Autodesk Inventor part; units mm, degrees
ref_plane "YZ Plane" through (0, 0, 0) normal (1, 0, 0) x (0, 1, 0)
ref_plane "XY Plane" through (0, 0, 0) normal (0, 0, 1) x (1, 0, 0)
sketch "Sketch1" plane through (0, 0, 0) normal (0, 0, 1) x (1, 0, 0)
  line L0 (-17.25, -31.85) -> (4.85, -31.85)
  line L1 (4.85, -31.85) -> (4.85, 0)
  arc A0 (4.85, 0) -> (0, 4.85) centre (0, 0) ccw
  line L2 (0, 4.85) -> (-12.4, 4.85)
  arc A1 (-12.4, 4.85) -> (-17.25, 0) centre (-12.4, 0) ccw
  line L3 (-17.25, 0) -> (-17.25, -31.85)
  circle A2 centre (-6.2, -6.5) radius 2.75
  circle A3 centre (-6.2, -17.15) radius 1.95
  arc A4 (1.9991, -27.9755) -> (1.0928, -27.0978) centre (2.55, -26.5) ccw
  arc A5 (1.0928, -27.0978) -> (1.9991, -27.9755) centre (-0.065, -29.2) ccw
  arc A6 (-13.4928, -27.0978) -> (-14.3991, -27.9755) centre (-14.95, -26.5) ccw
  arc A7 (-14.3991, -27.9755) -> (-13.4928, -27.0978) centre (-12.335, -29.2) ccw
  line L4 (9.85, -61.85) -> (-22.25, -61.85)
  line L5 (-22.25, -61.85) -> (-22.25, -21.85)
  line L6 (-22.25, -21.85) -> (9.85, -21.85)
  line L7 (9.85, -21.85) -> (9.85, -61.85)
  circle A8 centre (2.55, -26.5) radius 1.575
  circle A9 centre (-14.95, -26.5) radius 1.575
  point P0 (0, 0)
  point P1 (1.0928, -27.0978)
  point P2 (1.9991, -27.9755)
  point P3 (-17.25, -21.85)
  point P4 (4.85, -21.85)
  dimension "d2" = 5
  dimension "d3" = 5
  dimension "d12" = 10
  dimension "d13" = 40
extrude "Extrusion2" add sketch "Sketch1" along normal blind 5 contours L3 L6 L1 L0 | L0 L1 L6 L7 L4 L5 L3 | A5 A8 | A7 A9
sketch "Sketch2" plane through (0, 0, 0) normal (0, 0, -1) x (-1, 0, 0)
  line L0 (22.25, -21.85) -> (22.25, -61.85)
  line L1 (22.25, -61.85) -> (18.25, -61.85)
  line L2 (18.25, -61.85) -> (18.25, -21.85)
  line L3 (18.25, -21.85) -> (22.25, -21.85)
  line L4 (22.25, -21.85) -> (22.25, -61.85)
  line L5 (-9.85, -61.85) -> (-9.85, -21.85)
  line L6 (-9.85, -21.85) -> (22.25, -21.85)
  line L7 (-9.85, -61.85) -> (-5.85, -61.85)
  line L8 (-5.85, -61.85) -> (-5.85, -21.85)
  line L9 (-5.85, -21.85) -> (-9.85, -21.85)
  line L10 (-9.85, -21.85) -> (-9.85, -61.85)
  point P0 (0, 0)
  point P1 (-4.85, -21.85)
  point P2 (17.25, -21.85)
  point P3 (-9.85, -21.85)
  dimension "d8" = 4
  dimension "d9" = 4
extrude "Extrusion3" add sketch "Sketch2" along normal blind 20
sketch "Sketch3" plane through (0, 0, -20) normal (0, 0, -1) x (-1, 0, 0)
  circle A0 centre (-2.55, -26.5) radius 1.575
  circle A1 centre (14.95, -26.5) radius 1.575
  circle A2 centre (6.2, -6.5) radius 2.95
  line L0 (-43.9339, 5.041) -> (56.0661, 5.041)
  line L1 (-23.9339, -29.6) -> (-43.9339, 5.041)
  line L2 (36.0661, -29.6) -> (-23.9339, -29.6)
  line L3 (56.0661, 5.041) -> (36.0661, -29.6)
  line L4 (22.25, -61.85) -> (-9.85, -61.85)
  line L5 (-9.85, -61.85) -> (-9.85, -21.85)
  line L6 (22.25, -61.85) -> (-9.85, -61.85)
  line L7 (-9.85, -61.85) -> (-9.85, -30.6)
  line L8 (-9.85, -30.6) -> (22.25, -30.6)
  line L9 (22.25, -30.6) -> (22.25, -61.85)
  point P0 (0, 0)
  dimension "d14" = 1
extrude "Extrusion4" add sketch "Sketch3" along normal blind 5 contours L8 L9 L4 L5
sketch "Sketch4" plane through (0, 0, 5) normal (0, 0, 1) x (1, 0, 0)
  circle A0 centre (-6.2, -46.85) radius 11.05
  line L0 (-22.25, -21.85) -> (-22.25, -61.85)
  line L1 (-22.25, -61.85) -> (9.85, -61.85)
  point P0 (0, 0)
  dimension "d17" = 22.1
  dimension "d18" = 16.05
  dimension "d19" = 15
extrude "Extrusion5" cut sketch "Sketch4" against normal up to surface (5 mm away)
sketch "Sketch5" plane through (0, 0, -25) normal (0, 0, -1) x (-1, 0, 0)
  circle A0 centre (6.2, -46.85) radius 4.508
  circle A1 centre (6.2, -46.85) radius 15
  line L0 (22.25, -21.85) -> (22.25, -61.85)
  line L1 (22.25, -46.85) -> (-9.85, -46.85)
  line L2 (-9.85, -61.85) -> (-9.85, -21.85)
  line L3 (22.25, -46.85) -> (22.25, -61.85)
  line L4 (22.25, -61.85) -> (-9.85, -61.85)
  line L5 (-9.85, -46.85) -> (-9.85, -61.85)
  point P0 (0, 0)
  point P1 (6.2, -61.85)
  point P2 (21.2, -46.85)
  point P3 (-8.8, -46.85)
  dimension "d22" = 30
extrude "Extrusion6" cut sketch "Sketch5" against normal up to surface (30 mm away) contours L1 L0 L4 A1 | A1 L4 L2 L1
ref_plane "Work Plane1" through (-6.2, -61.85, -25) normal (0, 1, 0) x (-1, 0, 0)
sketch "Sketch6" plane through (-6.2, -61.85, -25) normal (0, 1, 0) x (-1, 0, 0)
  line L0 (-15, 0) -> (15, 0)
  line L1 (-15, 0) -> (-15, 30)
  line L2 (15, 30) -> (-15, 30)
  line L3 (15, 0) -> (15, 30)
  line L4 (12.05, 5) -> (-12.05, 5)
  line L5 (12.05, 25) -> (12.05, 5)
  line L6 (-12.05, 25) -> (12.05, 25)
  line L7 (-12.05, 5) -> (-12.05, 25)
  line L8 (-12.05, 25) -> (12.05, 25)
  line L9 (12.05, 25) -> (12.05, 26.5)
  line L10 (12.05, 26.5) -> (-12.05, 26.5)
  line L11 (-12.05, 26.5) -> (-12.05, 25)
  line L12 (-12.05, 5) -> (12.05, 5)
  line L13 (12.05, 5) -> (12.05, 3.5)
  line L14 (12.05, 3.5) -> (-12.05, 3.5)
  line L15 (-12.05, 3.5) -> (-12.05, 5)
  point P0 (-6.2, 25)
  dimension "d25" = 1.5
  dimension "d26" = 1.5
extrude "Extrusion7" cut sketch "Sketch6" along normal up to surface (40 mm away) contours L13 L14 L15 L4 | L6 L11 L10 L9
properties part number "arm1"
The listing builds one solid part. Answer for the finished solid, in the listing's coordinates (mm). A direction names the side the tool comes from. Give positions to 0.01 mm unless a question says otherwise; leave off trailing zeros. Write each loop counter-clockwise with the first axis right and the second up, starting at its lowest first coordinate (ties: lowest second). Pieces come first, ordered by that corner, then holes. Notation, with made-up numbers: M 40,2 L 97,2 A14 ccw 97,19 Z; hole C 81.5,52.25 d6. An arc over 180 degrees is marked long. Write each question's results on one line, items separated by ' | '.
Q1. Section C-C, the plane x = -15 is taken. Write down the section's boundary in (y, z), then the cut area to 3 significant figures.
Output values:
outline: M -59,-25 L -30.6,-25 L -30.6,-21.5 L -59,-21.5 Z; M -59,1.5 L -53.53,1.5 L -53.53,5 L -59,5 Z; M -40.17,1.5 L -28.07,1.5 L -28.07,5 L -40.17,5 Z; M -24.93,1.5 L -21.85,1.5 L -21.85,5 L -24.93,5 Z | area: 172 mm2
Q2. Section A-A, the plane z = -14.5 is taken. Write down the section's boundary in (x, y).
Output values:
outline: M -22.25,-46.85 L -21.2,-46.85 A15 ccw -18.25,-55.78 L -18.25,-21.85 L -22.25,-21.85 Z; M 5.85,-55.78 A15 ccw 8.8,-46.85 L 9.85,-46.85 L 9.85,-21.85 L 5.85,-21.85 Z
Q3. Section B-B, the plane x = -6.2 is taken. Write down the section's boundary in (y, z).
Output values:
outline: M -61.85,-25 L -30.6,-25 L -30.6,-21.5 L -61.85,-21.5 Z; M -61.85,1.5 L -57.9,1.5 L -57.9,5 L -61.85,5 Z; M -35.8,1.5 L -21.85,1.5 L -21.85,5 L -35.8,5 Z
Q4. Consider L1, parallel to X at y = -35, z = -17.75; L2, parallel to Y at x = -6.2, z = 3.5; L3, parallel to Z at x = -10, y = -32.5. Determine where each line is inside the solid, lowest interval first. Write a range as from..to.
Output values:
L1: -22.25..-18.25, 5.85..9.85 | L2: -61.85..-57.9, -35.8..-21.85 | L3: -25..-21.5, 1.5..5
Q5. Section D-D, the plane y = -46 is taken. Write down the section's boundary in (x, z).
Output values:
outline: M -22.25,-25 L 9.85,-25 L 9.85,5 L 4.82,5 L 4.82,1.5 L 5.85,1.5 L 5.85,-21.5 L -18.25,-21.5 L -18.25,1.5 L -17.22,1.5 L -17.22,5 L -22.25,5 Z
Q6. For a pull along Y with two mould halves and no side action, classify faces 1 (the flat face through (-22.25, -34, -10)), 2 (the cylindrical face through (-7.638, -35.894, 3.274)), 3 (the cylindrical face through (-16.088, -25.411, 3.226)), 4 (the flat face through (9, -46.85, -10)) as released by +Y, released by -Y, zero draft, split by the parting line, or undercut.
Output values:
face 1: zero draft | face 2: undercut | face 3: undercut | face 4: released by -Y
Q7. A tool of negligible diameter and unlimited length cuts with its end or side. For faces 5 (the flat face through (-22, -46.85, -10)), 6 (the flat face through (-20, -26, -20)), 7 (the flat face through (-6, -46, -21.5)), from which of +Z, -Z, +X, -X, +Y, -Y can it reach the whole face along a straight path? Write none if from no direction.
Output values:
face 5: +Z, -Z, -X, -Y | face 6: -Z, +X, -X, +Y | face 7: +Y, -Y
Q8. Flat-ended cylindrical pins translate along their axes: P1, Ø2, axis at x = -20, y = -26, coming from the -Z side; P2, Ø2, axis at x = 4.5, z = -21.5, coming from the -Y side; P3, Ø1, axis at x = -6, y = -29, coming from the -Z side; P4, Ø1.9, axis at x = -14.95, y = -26.5, coming from the -Z side. Find the tip coordinate at first contact, or state that the pin passes through.
Output values:
P1: z = -20 | P2: y = -58.29 | P3: z = 1.5 | P4: through
